Geometry check sheet. Reference: the model listing, model coordinates, mm. Coordinates: 2 decimals unless noted, no trailing zeros. Loops run counter-clockwise (first coordinate to the right, second up) from the corner with the lowest first, then second, coordinate; pieces in that order, holes last. Notation, with made-up numbers: M -23.5,62.25 L 6.5,62.25 A26 cw 6.5,86.25 Z; hole C 89,-25.5 d7. An arc over 180 degrees is marked long. Use CSV: the item, a comma, the result in double quotes.
```python
from build123d import *

# Parameters (mm, degrees)
PROFILE_1_R         = 3.25
PROFILE_1_R_2       = 6.25
PROFILE_1_R_3       = 1.65
PROFILE_1_R_4       = 2.2
WHEEL_CARRIER_DEPTH = 4
PIVOT_LANDS_START   = 4
PROFILE_2_R         = 3.25
PIVOT_LANDS_DEPTH   = 3
NUT_SEATS_C_D_START = -0.01
NUT_SEATS_C_D_DEPTH = 3.01


with BuildPart() as part:
    # Profile_1 → Wheel_carrier (new body)
    with BuildSketch(Plane.XY):
        Polygon((-12.750208645, 2.536174186), (-29.473182851, -101.712403875), (-29.473182851, -131.287596125), (-28.487699441, -133.666763538), (-26.666763538, -135.487699441), (-24.287596125, -136.473182851), (-4.291987084, -138.577276169), (4.291987084, -138.577276169), (24.287596125, -136.473182851), (26.666763538, -135.487699441), (28.487699441, -133.666763538), (29.473182851, -131.287596125), (29.473182851, -88.712403875), (12.750208645, 2.536174186), (10.80910496, 7.222413029), (7.222413029, 10.80910496), (2.536174186, 12.750208645), (-2.536174186, 12.750208645), (-7.222413029, 10.80910496), (-10.80910496, 7.222413029), align=None)
        Circle(PROFILE_1_R, mode=Mode.SUBTRACT)
        with Locations((0, -62)):
            Circle(PROFILE_1_R, mode=Mode.SUBTRACT)
        with Locations((0, -110)):
            Circle(PROFILE_1_R_2, mode=Mode.SUBTRACT)
        with Locations((15.5, -117)):
            Circle(PROFILE_1_R_3, mode=Mode.SUBTRACT)
        with Locations((7.75, -103.576606241)):
            Circle(PROFILE_1_R_3, mode=Mode.SUBTRACT)
        with Locations((-7.75, -103.576606241)):
            Circle(PROFILE_1_R_3, mode=Mode.SUBTRACT)
        with Locations((-15.5, -117)):
            Circle(PROFILE_1_R_3, mode=Mode.SUBTRACT)
        with Locations((-7.75, -130.423393759)):
            Circle(PROFILE_1_R_3, mode=Mode.SUBTRACT)
        with Locations((7.75, -130.423393759)):
            Circle(PROFILE_1_R_3, mode=Mode.SUBTRACT)
        with Locations((-23, -130)):
            Circle(PROFILE_1_R_4, mode=Mode.SUBTRACT)
        with Locations((23, -130)):
            Circle(PROFILE_1_R_4, mode=Mode.SUBTRACT)
        with Locations((-23, -103)):
            Circle(PROFILE_1_R_4, mode=Mode.SUBTRACT)
        with Locations((23, -90)):
            Circle(PROFILE_1_R_4, mode=Mode.SUBTRACT)
    extrude(amount=WHEEL_CARRIER_DEPTH)

    # Profile_2 → Pivot_lands (add)
    with BuildSketch(Plane.XY.offset(PIVOT_LANDS_START)):
        Polygon((12.750208645, -64.536174186), (12.750208645, 2.536174186), (10.80910496, 7.222413029), (7.222413029, 10.80910496), (2.536174186, 12.750208645), (-2.536174186, 12.750208645), (-7.222413029, 10.80910496), (-10.80910496, 7.222413029), (-12.750208645, 2.536174186), (-12.750208645, -64.536174186), (-10.80910496, -69.222413029), (-7.222413029, -72.80910496), (-2.536174186, -74.750208645), (2.536174186, -74.750208645), (7.222413029, -72.80910496), (10.80910496, -69.222413029), align=None)
        Circle(PROFILE_2_R, mode=Mode.SUBTRACT)
        with Locations((0, -62)):
            Circle(PROFILE_2_R, mode=Mode.SUBTRACT)
    extrude(amount=PIVOT_LANDS_DEPTH)

    # Profile_3 → Nut_seats_C_D (cut)
    with BuildSketch(Plane.XY.offset(NUT_SEATS_C_D_START)):
        Polygon((5.175, 2.987787643), (0, 5.975575286), (-5.175, 2.987787643), (-5.175, -2.987787643), (0, -5.975575286), (5.175, -2.987787643), align=None)
        Polygon((5.175, -59.012212357), (0, -56.024424714), (-5.175, -59.012212357), (-5.175, -64.987787643), (0, -67.975575286), (5.175, -64.987787643), align=None)
    extrude(amount=NUT_SEATS_C_D_DEPTH, mode=Mode.SUBTRACT)


solid = part.part
```
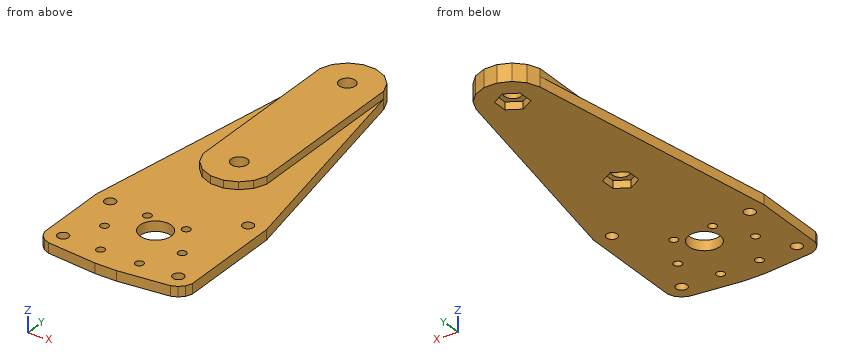
1. Section check C-C, the plane y = -12. Record the cut outline in (x, z).
The answers:
outline,"M -15.08,0 L 15.41,0 L 15.41,4 L 12.75,4 L 12.75,7 L -12.75,7 L -12.75,4 L -15.08,4 Z"
2. Thickness scan on line 1 (Y direction, x = 0, z = 1.1); line 2 (Y direction, x = 0, z = 4.95); line 3 (X direction, y = -2, z = 6.75). Record the ranges inside material, lowest first. Write a range as [from, to].
The answers:
line 1,"[-138.58, -116.25], [-103.75, -67.98], [-56.02, -5.98], [5.98, 12.75]"
line 2,"[-74.75, -65.25], [-58.75, -3.25], [3.25, 12.75]"
line 3,"[-12.75, -2.56], [2.56, 12.75]"
3. Gauge pin test, flat ends, axial feed: P1, Ø5, axis at x = 23, y = -130, coming from the +Z side; P2, Ø3.5, axis at y = -63, z = 2, coming from the -X side; P3, Ø3, axis at x = 7.75, y = -130.42, coming from the -Z side; P4, Ø1.5, axis at y = -1.5, z = 2, coming from the -X side. Record the tip position at first contact, or that the pin passes through.
The answers:
P1,"z = 4"
P2,"x = -23.54"
P3,"through"
P4,"x = -13.52"
4. Section check A-A, the plane x = 15.5. Record the cut outline in (y, z), plus the area to 3 significant figures.
The answers:
outline,"M -137.4,0 L -118.65,0 L -118.65,4 L -137.4,4 Z; M -115.35,0 L -12.47,0 L -12.47,4 L -115.35,4 Z"
area,"487 mm^2"
5. Section check B-B, the plane y = -43. Record the cut outline in (x, z).
The answers:
outline,"M -20.05,0 L 21.1,0 L 21.1,4 L 12.75,4 L 12.75,7 L -12.75,7 L -12.75,4 L -20.05,4 Z"
